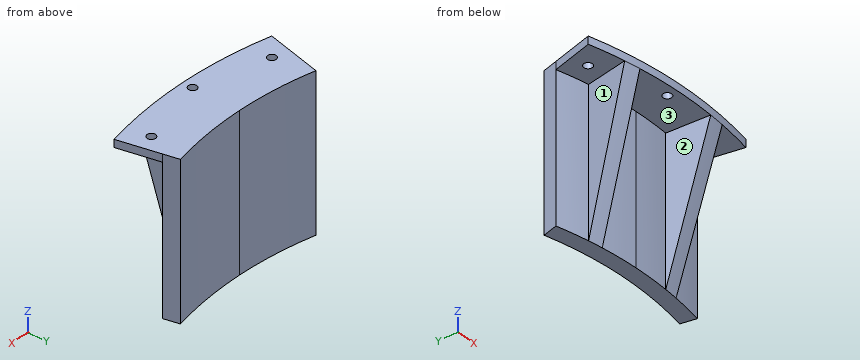
from build123d import *
from build123d.topology import SkipClean

# Parameters (mm, degrees)
EXTRUDE_1_DEPTH     = 60
EXTRUDE_START       = -3
EXTRUDE_2_DEPTH     = 3
EXTRUDE_START_2     = 57
SKETCH_3_R          = 1.65
EXTRUDE_3_DEPTH     = 57
SKETCH_4_R          = 1.65
CUT_EXTRUDE_1_DEPTH = 175.629425377


with BuildPart() as part:
    # 草图1 → 凸台-拉伸1 (new body)
    with BuildSketch(Plane.XY):
        with BuildLine():
            ThreePointArc((0, -143.5), (16.244661176, -142.57756129), (32.280476298, -139.822104297))
            Line((32.280476298, -139.822104297), (30.930769972, -133.975883908))
            ThreePointArc((30.930769972, -133.975883908), (15.565441893, -136.616130156), (0, -137.5))
            Line((0, -137.5), (0, -143.5))
        make_face()
        with BuildLine():
            Line((-30.930769972, -133.975883908), (-32.280476298, -139.822104297))
            ThreePointArc((-32.280476298, -139.822104297), (-16.244661176, -142.57756129), (0, -143.5))
            Line((0, -143.5), (0, -137.5))
            ThreePointArc((0, -137.5), (-15.565441893, -136.616130156), (-30.930769972, -133.975883908))
        make_face()
    extrude(amount=EXTRUDE_1_DEPTH)

    # 草图2 → 凸台-拉伸2 (add)
    with BuildSketch(Plane.XY.offset(60).offset(EXTRUDE_START)):
        with BuildLine():
            Line((35.992168695, -155.899210366), (32.280476298, -139.822104297))
            ThreePointArc((32.280476298, -139.822104297), (0, -143.5), (-32.280476298, -139.822104297))
            Line((-32.280476298, -139.822104297), (-35.992168695, -155.899210366))
            ThreePointArc((-35.992168695, -155.899210366), (0, -160), (35.992168695, -155.899210366))
        make_face()
    extrude(amount=EXTRUDE_2_DEPTH)

    # 草图3 → 凸台-拉伸3 (add)
    with SkipClean():  # the faces are left unmerged after this step: merging them gives an invalid solid
        with BuildSketch(Plane(origin=(0, 0, 57), x_dir=(-1, 0, 0), z_dir=(0, 0, -1)).offset(EXTRUDE_START_2)):
            with Locations(Location((-27.517564349, -148.471491042, 0), (0, 0, 180))):
                Circle(SKETCH_3_R)
            with Locations(Location((0, -156, 0), (0, 0, 180))):
                Circle(SKETCH_3_R)
            with BuildLine():
                Line((-16.169007549, -159.180913413), (-14.501578646, -142.765381717))
                ThreePointArc((-14.501578646, -142.765381717), (-17.239636373, -142.460678567), (-19.971339988, -142.103467864))
                Line((-19.971339988, -142.103467864), (-22.267696154, -158.442890999))
                ThreePointArc((-22.267696154, -158.442890999), (-19.221894214, -158.841174709), (-16.169007549, -159.180913413))
            make_face()
            with BuildLine():
                ThreePointArc((19.971339988, -142.103467864), (17.239636373, -142.460678567), (14.501578646, -142.765381717))
                Line((14.501578646, -142.765381717), (16.169007549, -159.180913413))
                ThreePointArc((16.169007549, -159.180913413), (19.221894214, -158.841174709), (22.267696154, -158.442890999))
                Line((22.267696154, -158.442890999), (19.971339988, -142.103467864))
            make_face()
            with Locations(Location((27.517564349, -148.471491042, 0), (0, 0, 180))):
                Circle(SKETCH_3_R)
        extrude(amount=-EXTRUDE_3_DEPTH)

    # 草图4 → 切除-拉伸1 (cut, through all)
    with SkipClean():  # the faces are left unmerged after this step: merging them gives an invalid solid
        with BuildSketch(Plane(origin=(0, 0, 0), x_dir=(-1, 0, 0), z_dir=(0, 0, -1))):
            with Locations((-27.517564349, -148.471491042)):
                Circle(SKETCH_4_R)
            with Locations((0, -156)):
                Circle(SKETCH_4_R)
            with Locations((27.517564349, -148.471491042)):
                Circle(SKETCH_4_R)
        extrude(amount=-CUT_EXTRUDE_1_DEPTH, mode=Mode.SUBTRACT)

    # 草图6 → 切除-旋转1 (revolve, cut)
    with BuildSketch(Plane(origin=(0, 0, 0), x_dir=(0, 0, -1), z_dir=(0.9902680687415703, 0.13917310096006566, 0))):
        Polygon((0, -143.5), (-57, -160), (0, -160), align=None)
    revolve(axis=Axis((0, 0, 60), (0, 0, -1)), mode=Mode.SUBTRACT)


solid = part.part
Check sheet for the modelled part. Datum: model origin and axes. Units: mm. Face numbers are marked on the shaded views. Round coordinates to 2 decimals unless told otherwise and drop trailing zeros. Loops run counter-clockwise (first coordinate to the right, second up) from the corner with the lowest first, then second, coordinate; pieces in that order, holes last. Notation, with made-up numbers: M -1.5,-17.5 L 16.5,-17.5 A22 ccw 16.5,-6.5 Z; hole C 54,-39 d9. An arc over 180 degrees is marked long. One line per item, written item: value.
(1) Sectioned sample at A-A, the plane z = 13. Record the cut outline in (x, y), then the cut area to 3 significant figures.
Computed values:
outline: M -32.28,-139.82 A143.5 ccw -19.97,-142.1 L -20.5,-145.83 A147.26 ccw -14.88,-146.51 L -14.5,-142.77 A143.5 ccw 14.5,-142.77 L 14.88,-146.51 A147.26 ccw 20.5,-145.83 L 19.97,-142.1 A143.5 ccw 32.28,-139.82 L 30.93,-133.98 A137.5 cw -30.93,-133.98 Z
area: 425 mm^2
(2) Sectioned sample at B-B, the plane x = 13. Record the cut outline in (y, z).
Computed values:
outline: M -159.47,57 L -142.91,57 L -142.91,0 L -136.88,0 L -136.88,60 L -159.47,60 Z
(3) Depth check by flat-ended pin: pin 1 Ø5.5 at (x, y) = (0, -156) entering from -Z; pin 2 Ø1 at (x, z) = (0, 24.5) entering from -Y; pin 3 Ø8 at (y, z) = (-141.5, 39) entering from -X; pin 4 Ø2 at (x, y) = (-27.52, -148.47) entering from +Z. Enter the tip coordinate at first touch or a pass-through.
Computed values:
pin 1: stops at z = 57
pin 2: stops at y = -143.5
pin 3: stops at x = -32.28
pin 4: passes through
(4) Sectioned sample at D-D, the plane x = 24. Record the cut outline in (y, z), then the cut area to 3 significant figures.
Computed values:
outline: M -158.19,57 L -141.48,57 L -141.48,0 L -135.39,0 L -135.39,60 L -158.19,60 Z
area: 416 mm^2
(5) Release check for a two-part mould opening along Y. For the marked faces 1, 2 and 3 record: +Y half, -Y half, draft (parallel to the pull), parting line (faces both ways), or undercut.
Computed values:
face 1: undercut
face 2: -Y half
face 3: draft
(6) Sectioned sample at C-C, the plane z = 43. Record the cut outline in (x, y), then the cut area to 3 significant figures.
Computed values:
outline: M -32.28,-139.82 A143.5 ccw -19.97,-142.1 L -21.7,-154.43 A155.95 ccw -15.76,-155.15 L -14.5,-142.77 A143.5 ccw 14.5,-142.77 L 15.76,-155.15 A155.95 ccw 21.7,-154.43 L 19.97,-142.1 A143.5 ccw 32.28,-139.82 L 30.93,-133.98 A137.5 cw -30.93,-133.98 Z
area: 526 mm^2
(7) Thickness scan on line 1 (Z direction, x = -15.5, y = -154); line 2 (X direction, y = -149, z = 47); line 3 (X direction, y = -147.75, z = 32.5). Record the ranges inside material, lowest first.
Computed values:
line 1: z = 57 to 60
line 2: x = -20.94 to -15.13, 15.13 to 20.94
line 3: x = -20.76 to -15.01, 15.01 to 20.76
